from build123d import *

# Parameters (mm, degrees)
BOSS_EXTRUDE1_DEPTH = 5
SKETCH2_R           = 2
CUT_EXTRUDE1_DEPTH  = 4
FILLET1_R           = 4
FILLET2_R           = 2


with BuildPart() as part:
    # Sketch1 → Boss-Extrude1 (new body, symmetric)
    with BuildSketch(Plane.XY):
        with BuildLine():
            Line((-5.5, -2.5), (-5.5, 0))
            ThreePointArc((-5.5, 0), (0, 5.5), (5.5, 0))
            Line((5.5, 0), (5.5, -2.5))
            Line((5.5, -2.5), (8.124038405, -2.5))
            ThreePointArc((8.124038405, -2.5), (8.405484116, -1.264055687), (8.5, 0))
            ThreePointArc((8.5, 0), (0, 8.5), (-8.5, 0))
            ThreePointArc((-8.5, 0), (-8.405484116, -1.264055687), (-8.124038405, -2.5))
            Line((-8.124038405, -2.5), (-5.5, -2.5))
        make_face()
        with BuildLine():
            Line((-5.5, -5.5), (-5.5, -2.5))
            Line((-5.5, -2.5), (-8.124038405, -2.5))
            ThreePointArc((-8.124038405, -2.5), (-7.454857018, -4.083516479), (-6.480740698, -5.5))
            Line((-6.480740698, -5.5), (-5.5, -5.5))
        make_face()
        with BuildLine():
            ThreePointArc((-6.480740698, -5.5), (-7.454857018, -4.083516479), (-8.124038405, -2.5))
            Line((-8.124038405, -2.5), (-8.5, -2.5))
            Line((-8.5, -2.5), (-20, -2.5))
            Line((-20, -2.5), (-20, -5.5))
            Line((-20, -5.5), (-6.480740698, -5.5))
        make_face()
        with BuildLine():
            Line((8.124038405, -2.5), (5.5, -2.5))
            Line((5.5, -2.5), (5.5, -5.5))
            Line((5.5, -5.5), (6.480740698, -5.5))
            ThreePointArc((6.480740698, -5.5), (7.454857018, -4.083516479), (8.124038405, -2.5))
        make_face()
        with BuildLine():
            Line((8.5, -2.5), (8.124038405, -2.5))
            ThreePointArc((8.124038405, -2.5), (7.454857018, -4.083516479), (6.480740698, -5.5))
            Line((6.480740698, -5.5), (20, -5.5))
            Line((20, -5.5), (20, -2.5))
            Line((20, -2.5), (8.5, -2.5))
        make_face()
        with BuildLine():
            ThreePointArc((8.5, 0), (8.405484116, -1.264055687), (8.124038405, -2.5))
            Line((8.124038405, -2.5), (8.5, -2.5))
            Line((8.5, -2.5), (8.5, 0))
        make_face()
        with BuildLine():
            Line((-8.5, -2.5), (-8.124038405, -2.5))
            ThreePointArc((-8.124038405, -2.5), (-8.405484116, -1.264055687), (-8.5, 0))
            Line((-8.5, 0), (-8.5, -2.5))
        make_face()
    extrude(amount=BOSS_EXTRUDE1_DEPTH, both=True)

    # Sketch2 → Cut-Extrude1 (cut, through all)
    with BuildSketch(Plane(origin=(0, -2.5, 0), x_dir=(1, 0, 0), z_dir=(0, 1, 0))):
        with Locations((-15, 0)):
            Circle(SKETCH2_R)
        with Locations((15, 0)):
            Circle(SKETCH2_R)
    extrude(amount=-CUT_EXTRUDE1_DEPTH, mode=Mode.SUBTRACT)

    # Fillet1
    fillet1_edges = [part.edges().sort_by_distance(p)[0] for p in [
        (20, -4, -5),
        (-20, -4, -5),
        (-20, -4, 5),
        (20, -4, 5),
    ]]
    fillet(fillet1_edges, radius=FILLET1_R)

    # Fillet2
    fillet2_edges = [part.edges().sort_by_distance(p)[0] for p in [
        (-8.5, -2.5, 0),
        (8.5, -2.5, 0),
    ]]
    fillet(fillet2_edges, radius=FILLET2_R)


solid = part.part
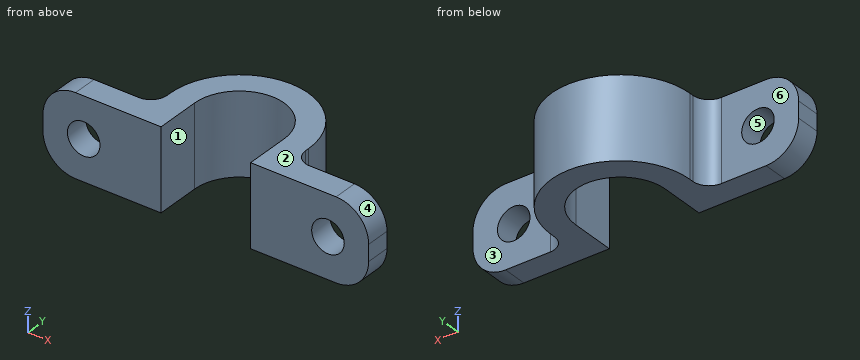
Verification items for the finished model (mm, model axes). Face numbers are marked on the shaded views. A direction names the side the tool comes from. Coordinates: 2 decimals unless noted, no trailing zeros. Write each loop counter-clockwise with the first axis right and the second up, starting at its lowest first coordinate (ties: lowest second). Pieces come first, ordered by that corner, then holes. Notation, with made-up numbers: M -24,-33 L 27,-33 A21 ccw 27,-19 Z; hole C 37,55 d2. An arc over 180 degrees is marked long. Use a Markdown table: item, result.
Q1. Thickness scan on line 1 (X direction, y = -4.75, z = 0); line 2 (Y direction, x = 0, z = 3.5); line 3 (X direction, y = 3.75, z = 2.5). Record the ranges inside material, lowest first.
Reply:
| item | result |
|---|---|
| line 1 | x = -20 to -17, -13 to -5.5, 5.5 to 13, 17 to 20 |
| line 2 | y = 5.5 to 8.5 |
| line 3 | x = -7.63 to -4.02, 4.02 to 7.63 |
Q2. Sectioned sample at C-C, the plane z = 0. Record the boundary of the cut face in (x, y), plus the area to 3 significant figures.
Reply:
| item | result |
|---|---|
| outline | M -20,-5.5 L -17,-5.5 L -17,-2.5 L -20,-2.5 Z; M -13,-5.5 L -5.5,-5.5 L -5.5,0 A5.5 cw 5.5,0 L 5.5,-5.5 L 13,-5.5 L 13,-2.5 L 10.5,-2.5 A2 cw 8.5,-0.5 L 8.5,0 A8.5 ccw -8.5,0 L -8.5,-0.5 A2 cw -10.5,-2.5 L -13,-2.5 Z; M 17,-5.5 L 20,-5.5 L 20,-2.5 L 17,-2.5 Z |
| area | 146 mm² |
Q3. Sectioned sample at A-A, the plane y = -4. Record the boundary of the cut face in (x, z), plus the area to 3 significant figures.
Reply:
| item | result |
|---|---|
| outline | M -20,-1 A4 ccw -16,-5 L -5.5,-5 L -5.5,5 L -16,5 A4 ccw -20,1 Z; M 5.5,-5 L 16,-5 A4 ccw 20,-1 L 20,1 A4 ccw 16,5 L 5.5,5 Z; hole C -15,0 d4; hole C 15,0 d4 |
| area | 251 mm² |
Q4. Go/stop test with flat-tipped pins: P1, Ø0.6, axis at y = 0, z = -1.5, coming from the -X side; P2, Ø3.5, axis at x = 15, z = 0, coming from the +Y side; P3, Ø6, axis at x = 13.5, z = -3, coming from the +Y side; P4, Ø2, axis at y = 5, z = 1, coming from the -X side. Record where each tip stops, or that it passes through.
Reply:
| item | result |
|---|---|
| P1 | stops at x = -8.5 |
| P2 | passes through |
| P3 | stops at y = -2.5 |
| P4 | stops at x = -7.5 |
Q5. Sectioned sample at D-D, the plane y = -1.75. Record the boundary of the cut face in (x, z), plus the area to 3 significant figures.
Reply:
| item | result |
|---|---|
| outline | M -8.94,-5 L -5.5,-5 L -5.5,5 L -8.94,5 Z; M 5.5,-5 L 8.94,-5 L 8.94,5 L 5.5,5 Z |
| area | 68.8 mm² |
Q6. Set-up check for the marked faces 1, 2 and 3: record each of +Z, -Z, +X, -X, +Y, -Y from which the full face is reachable in a straight line by a thin tool's end or side.
Reply:
| item | result |
|---|---|
| face 1 | +Z, -Z, -Y |
| face 2 | +Z, +X, -X, +Y, -Y |
| face 3 | +Z, -Z, +X, +Y |
Q7. Draft check along Z on the marked faces 4, 5 and 6. Enter one of: +Z half, -Z half, draft (parallel to the pull), parting line (faces both ways), or undercut.
Reply:
| item | result |
|---|---|
| face 4 | +Z half |
| face 5 | undercut |
| face 6 | draft |
Q8. Sectioned sample at B-B, the plane x = 15. Record the boundary of the cut face in (y, z), plus the area to 3 significant figures.
Reply:
| item | result |
|---|---|
| outline | M -5.5,-5 L -2.5,-5 L -2.5,-2 L -5.5,-2 Z; M -5.5,2 L -2.5,2 L -2.5,5 L -5.5,5 Z |
| area | 18.0 mm² |
